Read the model definition and answer for the solid it produces. Units are mm, in the model's axes. Face numbers are marked on the shaded views. A direction names the side the tool comes from. Coordinates: 2 decimals unless noted, no trailing zeros. Loops run counter-clockwise (first coordinate to the right, second up) from the corner with the lowest first, then second, coordinate; pieces in that order, holes last.
from build123d import *

# Parameters (mm, degrees)
BOSS_EXTRUDE1_DEPTH = 20
SKETCH2_W           = 36
SKETCH2_H           = 20
CUT_EXTRUDE1_DEPTH  = 107.88908334
CUT_EXTRUDE3_DEPTH  = 10
CUT_EXTRUDE5_DEPTH  = 10
SKETCH6_R           = 19
SKETCH6_R_2         = 10
BOSS_EXTRUDE2_DEPTH = 20
CUT_EXTRUDE6_DEPTH  = 102.120107483
BOSS_EXTRUDE3_START = -26
BOSS_EXTRUDE3_DEPTH = 10
SKETCH9_R           = 5
CUT_EXTRUDE7_DEPTH  = 106.703210108


with BuildPart() as part:
    # Sketch1 → Boss-Extrude1 (new, symmetric)
    with BuildSketch(Plane.XY):
        Polygon((38, -89.784609691), (38, -25.784609691), (42, -25.784609691), (42, -20.784609691), (30, 0), (-30, 0), (-42, -20.784609691), (-42, -25.784609691), (-38, -25.784609691), (-38, -89.784609691), align=None)
    extrude(amount=BOSS_EXTRUDE1_DEPTH, both=True)

    # Sketch2 → Cut-Extrude1 (cut, through all)
    with BuildSketch(Plane.XY.offset(20)):
        with Locations((0, -79.784609691)):
            Rectangle(SKETCH2_W, SKETCH2_H)
    extrude(amount=-CUT_EXTRUDE1_DEPTH, mode=Mode.SUBTRACT)

    # Sketch3 → Cut-Extrude3 (cut)
    with BuildSketch(Plane.XY.offset(20)):
        with BuildLine():
            Line((-27, 0), (27, 0))
            ThreePointArc((27, 0), (0, -27), (-27, 0))
        make_face()
    extrude(amount=-CUT_EXTRUDE3_DEPTH, mode=Mode.SUBTRACT)

    # Sketch5 → Cut-Extrude5 (cut)
    with BuildSketch(Plane.XY.offset(10)):
        with BuildLine():
            Line((-19, 0), (19, 0))
            ThreePointArc((19, 0), (0, -19), (-19, 0))
        make_face()
    extrude(amount=-CUT_EXTRUDE5_DEPTH, mode=Mode.SUBTRACT)

    # Sketch6 → Boss-Extrude2 (add)
    with BuildSketch(Plane.XY):
        Circle(SKETCH6_R)
        Circle(SKETCH6_R_2, mode=Mode.SUBTRACT)
    extrude(amount=-BOSS_EXTRUDE2_DEPTH)

    # Sketch6<2> → Cut-Extrude6 (cut, through all)
    with BuildSketch(Plane.XY):
        with BuildLine():
            Line((-10, 0), (10, 0))
            ThreePointArc((10, 0), (0, 10), (-10, 0))
        make_face()
        with BuildLine():
            ThreePointArc((-10, 0), (0, -10), (10, 0))
            Line((10, 0), (-10, 0))
        make_face()
    extrude(amount=-CUT_EXTRUDE6_DEPTH, mode=Mode.SUBTRACT)

    # Sketch8 → Boss-Extrude3 (add)
    with BuildSketch(Plane(origin=(0, 0, 0), x_dir=(1, 0, 0), z_dir=(0, 1, 0)).offset(BOSS_EXTRUDE3_START)):
        with BuildLine():
            Line((63, 10), (27, 10))
            Line((27, 10), (27, -10))
            Line((27, -10), (63, -10))
            ThreePointArc((63, -10), (73, 0), (63, 10))
        make_face()
    boss_extrude3 = extrude(amount=BOSS_EXTRUDE3_DEPTH)

    # Mirror1: Boss-Extrude3 across plane
    add(boss_extrude3.mirror(Plane(origin=(0, 0, 0), x_dir=(0, 0, 1), z_dir=(1, 0, 0))))

    # Sketch9 → Cut-Extrude7 (cut, through all)
    with BuildSketch(Plane(origin=(0, -16, 0), x_dir=(1, 0, 0), z_dir=(0, 1, 0))):
        with Locations(Location((-63, 0, 0), (0, 0, 270))):
            Circle(SKETCH9_R)
    cut_extrude7 = extrude(amount=-CUT_EXTRUDE7_DEPTH, mode=Mode.SUBTRACT)

    # Mirror2: Cut-Extrude7 across plane
    add(cut_extrude7.mirror(Plane(origin=(0, 0, 0), x_dir=(0, 0, 1), z_dir=(1, 0, 0))), mode=Mode.SUBTRACT)


solid = part.part
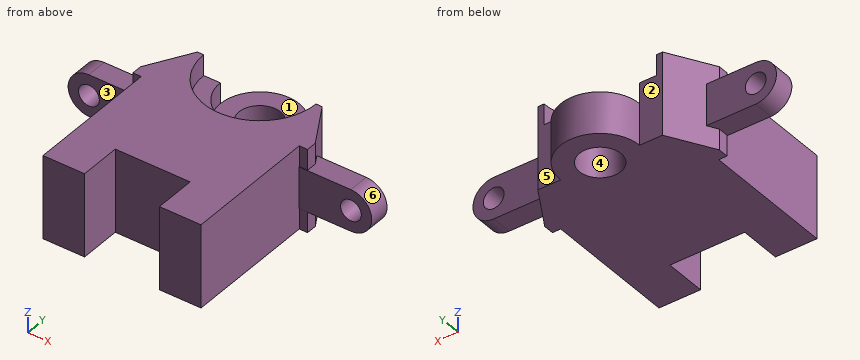
Item 1: Determine the mould class of the marked faces 4, 5 and 6 for opening direction X: released by +X, released by -X, zero draft, split by the parting line, or undercut.
Numbers:
face 4: undercut
face 5: zero draft
face 6: released by +X
Item 2: Which of the six approach directions +Z, -Z, +X, -X, +Y, -Y give full straight-line access (tool end or side, diameter ignored) to the marked faces 1, 2 and 3?
Numbers:
face 1: +Z, +Y
face 2: +Z, -Z, -X, +Y
face 3: +Z, -Z, -X, -Y
Item 3: A cutting plane is placed at C-C on y = 4.5. Determine the outline of the cut face in (x, z), then the cut area to 3 significant figures.
Numbers:
outline: (-18.46, -20) - (-8.93, -20) - (-8.93, 0) - (-18.46, 0) - close; (8.93, -20) - (18.46, -20) - (18.46, 0) - (8.93, 0) - close
area: 381 mm2
Item 4: A cutting plane is placed at A-A on z = -11.5. Determine the outline of the cut face in (x, y).
Numbers:
outline: (-42, -25.78) - (-38, -25.78) - (-38, -89.78) - (-18, -89.78) - (-18, -69.78) - (18, -69.78) - (18, -89.78) - (38, -89.78) - (38, -25.78) - (42, -25.78) - (42, -20.78) - (30, 0) - (19, 0) arc R19 ccw to (-19, 0) - (-30, 0) - (-42, -20.78) - close; hole circle Ø20 at (0, 0)
Item 5: Find the intervals of material crossed by line 1 along X through (y, z) = (-19.25, 0); line 2 along Y through (x, z) = (0, -12.25); line 3 along X through (y, z) = (-49.5, -12.5), in increasing order.
Numbers:
line 1: x = -73 to -68, -58 to 58, 68 to 73
line 2: y = -69.78 to -10, 10 to 19
line 3: x = -38 to 38
Item 6: A cutting plane is placed at B-B on x = 0. Determine the outline of the cut face in (y, z), then the cut area to 3 significant figures.
Numbers:
outline: (-69.78, -20) - (-10, -20) - (-10, 0) - (-19, 0) - (-19, 10) - (-27, 10) - (-27, 20) - (-69.78, 20) - close; (10, -20) - (19, -20) - (19, 0) - (10, 0) - close
area: 2,310 mm2
Item 7: A cutting plane is placed at D-D on z = 17. Determine the outline of the cut face in (x, y).
Numbers:
outline: (-42, -25.78) - (-38, -25.78) - (-38, -89.78) - (-18, -89.78) - (-18, -69.78) - (18, -69.78) - (18, -89.78) - (38, -89.78) - (38, -25.78) - (42, -25.78) - (42, -20.78) - (30, 0) - (27, 0) arc R27 cw to (-27, 0) - (-30, 0) - (-42, -20.78) - close
Item 8: Given pin 1 (4 mm diameter, centred on x = -2, z = -12.5, fed in from -Y); pin 2 (2.5 mm diameter, centred on y = -23.5, z = -14, fed in from +X); pin 3 (12 mm diameter, centred on y = -37.5, z = -11, fed in from +X), each flat-ended and moving along its own axis, determine where each tip first touches the part or whether it passes through.
Numbers:
pin 1: stops at y = -69.78
pin 2: stops at x = 42
pin 3: stops at x = 38
